Autodesk Inventor part; units mm, degrees
ref_plane "YZ Plane" through (0, 0, 0) normal (1, 0, 0) x (0, 1, 0)
ref_plane "XZ Plane" through (0, 0, 0) normal (0, 1, 0) x (-1, 0, 0)
ref_plane "XY Plane" through (0, 0, 0) normal (0, 0, 1) x (1, 0, 0)
sketch "Sketch1" plane through (0, 0, 0) normal (0, 1, 0) x (-1, 0, 0)
  line L0 (0, 0) -> (0, -244.423)
  line L1 (0, 0) -> (244.423, 0) construction
  line L2 (0, -244.423) -> (0, -285.4289)
  line L3 (0, -285.4289) -> (0, -529.8519)
  circle A0 centre (0, -244.423) radius 2.75
  circle A1 centre (0, -285.4289) radius 2.75
  circle A2 centre (0, 0) radius 2.75
  circle A3 centre (0, 0) radius 7.5
  circle A4 centre (0, -529.8519) radius 7.5
  circle A5 centre (0, -264.9259) radius 9
  spline S0 degree 2 poles (7.5, 0) (10.5, -264.9259) (7.5, -529.8519) knots 0 0 0 1 1 1
  spline S1 degree 2 poles (-7.5, -529.8519) (-10.5, -264.9259) (-7.5, 0) knots 0 0 0 1 1 1
  ellipse E0 centre (0, -264.9259) end of major axis (0, -104.9259) minor radius 2.7588
  circle A6 centre (0, -529.8519) radius 2.75
  circle A7 centre (0, -244.423) radius 7.5
  circle A8 centre (0, -285.4289) radius 7.5
  line L4 (7.5, -285.4289) -> (-7.5, -285.4289)
  line L5 (7.5, -244.423) -> (-7.5, -244.423)
  point P0 (9, -264.9259)
  point P1 (-9, -264.9259)
  point P2 (0, -522.3519)
  point P3 (0, -7.5)
  point P4 (-2.7354, -244.1399)
  point P5 (2.7354, -244.1399)
  point P6 (2.7366, -244.694)
  point P7 (2.7548, -256.3579)
  point P8 (-2.7548, -256.3579)
  point P9 (-2.7366, -244.694)
  point P10 (2.7548, -273.494)
  point P11 (2.7366, -285.1579)
  point P12 (2.7354, -285.712)
  point P13 (-2.7354, -285.712)
  point P14 (-2.7366, -285.1579)
  point P15 (-2.7548, -273.494)
  point P16 (2.7489, -278.4508)
  point P17 (-2.7489, -278.4508)
  point P18 (2.7489, -251.4011)
  point P19 (-2.7489, -251.4011)
  dimension "d15" = 160
  dimension "d0" = 244.423
  dimension "d1" = 90
  dimension "d2" = 41.0059
  dimension "d3" = 244.423
  dimension "d4" = 5.5
  dimension "d5" = 5.5
  dimension "d6" = 5.5
  dimension "d7" = 15
  dimension "d8" = 15
  dimension "d9" = 18
  dimension "d10" = 5.5
  dimension "d16" = 15
  dimension "d17" = 15
extrude "Extrusion1" add sketch "Sketch1" along normal blind 2 contours A3 | A4
extrude "Extrusion2" add sketch "Sketch1" along normal blind 1 contours A3 S0 A5 E0 A7 L0 | L0 E0 A7 A5 S1 A3 | E0 A0 L5 A7 | A7 L5 A0 E0 | A5 E0 | A5 E0 A8 L3 A4 S1 | A5 E0 | S0 A4 L3 E0 A8 A5 | L5 A0 E0 A7 | A7 E0 A0 L5 | E0 A1 L4 A8 | A8 L4 A1 E0 | L4 A1 E0 A8 | A8 E0 A1 L4
extrude "Extrusion3" add sketch "Sketch1" along normal blind 1 contours E0 A0 L2 A7 | A7 L2 A0 E0 | A8 L2 A1 E0 | E0 A1 L2 A8
properties part number "szalag3"
Could you check a few things on this model? Use its own coordinates, in mm. A direction names the side the tool comes from. Give positions to 0.01 mm unless a question says otherwise; leave off trailing zeros. Answer as CSV lines item,"result". Start each with the question number.
(1) If we section it at A-A, the plane y = 0.5: Give the number of separate pieces and of enclosed holes in the cut face, and give its area (3 significant figures).
(2) I'm going to push flat-ended pins straight in: pin 1 Ø6.5 at (x, z) = (0, -285.43) entering from +Y; pin 2 Ø1 at (x, y) = (5.5, 1.5) entering from -Z. Where does each tip first touch, or does it pass through?
(3) Please list where these lines run through material, in increasing order: line 1 (Z direction, x = 1.5, y = 1.15); line 2 (X direction, y = 0.9, z = 0); line 3 (X direction, y = 0.6, z = -288).
(4) Which directions (+Z, -Z, +X, -X, +Y, -Y) give clear straight access to the entire face, cutting with the end or side of a thin tool? Please do faces 1 (the face through (1.63, 1.21, 7.32)), 2 (the face through (4, 0, -261)).
Answer list:
1,separate pieces,"1"
1,enclosed holes,"5"
1,area,"7,810 mm^2"
2,pin 1,"y = 1"
2,pin 2,"z = -535.44"
3,line 1,"-537.2 to -532.16, -527.55 to -522.5, -7.35 to -2.3, 2.3 to 7.35"
3,line 2,"-7.5 to -2.75, 2.75 to 7.5"
3,line 3,"-8.99 to -2.73, 2.73 to 8.99"
4,face 1,"+Y"
4,face 2,"+Z, -Z, +X, -X, -Y"
